Here's how the part is built. I have some questions about the finished solid (model axes, mm). Round coordinates to 2 decimals unless told otherwise and drop trailing zeros. Write each loop counter-clockwise with the first axis right and the second up, starting at its lowest first coordinate (ties: lowest second). Pieces come first, ordered by that corner, then holes. Notation, with made-up numbers: (43, 1) -> (59, 1) arc R13 cw to (59, 8) -> close; hole circle Ø5 at (18, 66). An arc over 180 degrees is marked (long way). Answer in a Markdown table with one row per item.
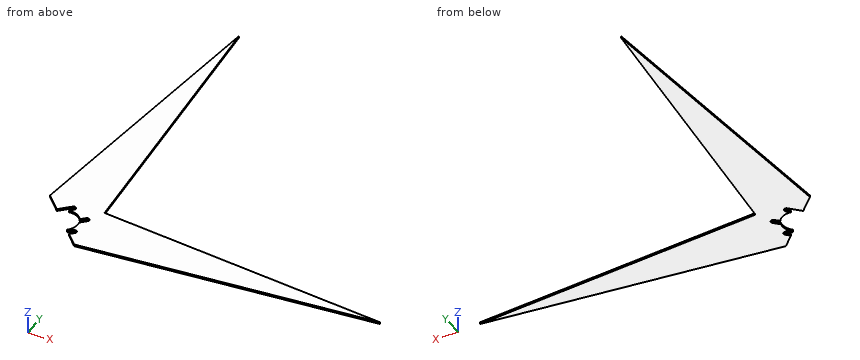
from build123d import *

# Parameters (mm, degrees)
SKETCH_1_R          = 2.6
SKETCH_1_R_2        = 17
EXTRUDE_1_DEPTH     = 2
CUT_EXTRUDE_2_DEPTH = 2


with BuildPart() as part:
    # 草图1 → 凸台-拉伸1 (new body)
    with BuildSketch(Plane.XY):
        Polygon((53.57, -53.57), (373.57, -23.57), (53.57, 6.43), (23.57, 326.43), (-6.43, 6.43), (-6.43, -53.57), align=None)
        with Locations((23.57, -47.32)):
            Circle(SKETCH_1_R, mode=Mode.SUBTRACT)
        with Locations((3.00189666, -11.695)):
            Circle(SKETCH_1_R, mode=Mode.SUBTRACT)
        with Locations((44.13810334, -11.695)):
            Circle(SKETCH_1_R, mode=Mode.SUBTRACT)
        with Locations((43.055571585, -34.82)):
            Circle(SKETCH_1_R, mode=Mode.SUBTRACT)
        with Locations((4.084428415, -34.82)):
            Circle(SKETCH_1_R, mode=Mode.SUBTRACT)
        with Locations((23.57, -1.07)):
            Circle(SKETCH_1_R, mode=Mode.SUBTRACT)
        with Locations((23.57, -23.57)):
            Circle(SKETCH_1_R_2, mode=Mode.SUBTRACT)
    extrude(amount=EXTRUDE_1_DEPTH)

    # 草图2 → 切除-拉伸2 (cut)
    with BuildSketch(Plane.XY.offset(2)):
        Polygon((53.57, -53.57), (-6.43, -53.57), (-6.43, 6.43), (10.481522369, -10.481522369), (21.731522369, 0.768477631), (25.408477631, -2.908477631), (14.158477631, -14.158477631), (26.078074039, -26.078074039), (42.299625709, -9.856522369), (45.976580971, -13.533477631), (29.755029301, -29.755029301), (37.099308161, -37.099308161), (41.217093954, -32.981522369), (44.894049216, -36.658477631), (40.776263424, -40.776263424), align=None)
    extrude(amount=-CUT_EXTRUDE_2_DEPTH, mode=Mode.SUBTRACT)


solid = part.part
1) I want a section at C-C, the plane y = 265.5. List the corners of the cut face in (x, z) for me.
Response:
| item | result |
|---|---|
| outline | (17.86, 0) -> (29.28, 0) -> (29.28, 2) -> (17.86, 2) -> close |
2) I need wall thicknesses on line 1 (Y direction, x = 209, z = 0.1); line 2 (X direction, y = 273.5, z = 1.2); line 3 (X direction, y = 240, z = 1.7). Which ranges of each line are inside material? Lowest first, please. Write a range as [from, to].
Response:
| item | result |
|---|---|
| line 1 | y = [-39, -8.14] |
| line 2 | x = [18.61, 28.53] |
| line 3 | x = [15.47, 31.67] |
3) I want a section at A-A, the plane z = 1.2. List the corners of the cut face in (x, y) for me (3 decimals), and give its area (3 significant figures).
Response:
| item | result |
|---|---|
| outline | (-6.43, 6.43) -> (10.482, -10.482) -> (21.732, 0.768) arc R2.6 cw to (25.408, -2.908) -> (21.637, -6.68) arc R17 cw to (37.834, -14.322) -> (42.3, -9.857) arc R2.6 cw to (45.977, -13.533) -> (40.063, -19.447) arc R17 cw to (35.591, -35.591) -> (37.099, -37.099) -> (41.217, -32.982) arc R2.6 cw to (44.894, -36.658) -> (40.776, -40.776) -> (53.57, -53.57) -> (373.57, -23.57) -> (53.57, 6.43) -> (23.57, 326.43) -> close |
| area | 20,400 mm^2 |
4) I want a section at B-B, the plane x = 225. List the corners of the cut face in (y, z) for me, and give its area (3 significant figures).
Response:
| item | result |
|---|---|
| outline | (-37.5, 0) -> (-9.64, 0) -> (-9.64, 2) -> (-37.5, 2) -> close |
| area | 55.7 mm^2 |
